Here's how the part is built. I have some questions about the finished solid (model axes, mm). A direction names the side the tool comes from. Round coordinates to 2 decimals unless told otherwise and drop trailing zeros. Loops run counter-clockwise (first coordinate to the right, second up) from the corner with the lowest first, then second, coordinate; pieces in that order, holes last. Notation, with made-up numbers: M -23,2 L 8,2 A15 cw 8,13 Z; hole C -37.75,-2.5 d5. An arc over 180 degrees is marked long. Answer as a JSON object with one key per item and string values.
from build123d import *

# Parameters (mm, degrees)
F1_DEPTH = 64.77
F3_DEPTH = 6.096
F4_R     = 5.860141
F5_DEPTH = 79.248


with BuildPart() as f1:
    # F0 (on Front) → F1 (new body)
    with BuildSketch(Plane.XZ):
        Polygon((32.464709, -14.754961), (0, 14.754961), (-32.464709, 14.754961), (-32.464709, -14.754961), align=None)
    extrude(amount=F1_DEPTH)

    # F2 (on Front) → F3 (join)
    with BuildSketch(Plane.XZ):
        Polygon((-32.523151, -14.200249), (42.600743, -14.200249), (0, 24.277844), (-32.523151, 24.277844), align=None)
    extrude(amount=-F3_DEPTH)

    # F4 (on face) → F5 (cut)
    with BuildSketch(Plane(origin=(0, 0, -14.754961), x_dir=(1, 0, 0), z_dir=(0, 0, -1))):
        with Locations((18.379251, 32.672778)):
            Circle(F4_R)
    extrude(amount=-F5_DEPTH, mode=Mode.SUBTRACT)


solid = f1.part
Item 1: If I drill on L1, parallel to Z at x = -19.5, y = -41; L2, parallel to Y at x = 1, z = 17; L3, parallel to Z at x = 20, y = -44.5, over which ranges is the centre line in solid material (lowest first)? Write a range as from..to.
Solution:
{"L1": "z = -14.75..14.75", "L2": "y = 0..6.1", "L3": "z = -14.75..-3.42"}
Item 2: I want a section at C-C on y = -54.5. List the corners of the cut face in (x, z) for me.
Solution:
{"outline": "M -32.46,-14.75 L 32.46,-14.75 L 0,14.75 L -32.46,14.75 Z"}
Item 3: I want a section at A-A on x = 20. List the corners of the cut face in (y, z) for me, plus the area to 3 significant figures.
Solution:
{"outline": "M -64.77,-14.75 L -38.3,-14.75 L -38.3,-3.42 L -64.77,-3.42 Z; M -27.04,-14.75 L 0,-14.75 L 0,-14.2 L 6.1,-14.2 L 6.1,6.21 L 0,6.21 L 0,-3.42 L -27.04,-3.42 Z", "area": "731 mm2"}
Item 4: For faces 1 (the face through (0, -32, -14.755)), 2 (the face through (16.46, -24.735, -0.207)), 3 (the face through (-16, -32, 14.755)), 4 (the face through (5, 3, -14.2)), 5 (the face through (-8, -64.77, 0)), which set-ups out of +Z, -Z, +X, -X, +Y, -Y let a thin tool reach every point of the face, with its end or its side?
Solution:
{"face 1": "-Z, +X, -X, +Y, -Y", "face 2": "+Z, +X, -Y", "face 3": "+Z, +X, -X, -Y", "face 4": "-Z, +X, -X, +Y", "face 5": "+Z, -Z, +X, -X, -Y"}
Item 5: I want a section at B-B on z = -11.5. List the corners of the cut face in (x, y) for me.
Solution:
{"outline": "M -32.52,0 L -32.46,0 L -32.46,-64.77 L 28.88,-64.77 L 28.88,0 L 39.61,0 L 39.61,6.1 L -32.52,6.1 Z; hole C 18.38,-32.67 d11.72"}
Item 6: For P1, Ø1.8, axis at x = 1.5, y = 1.5, coming from the -Z side; P2, Ø12, axis at y = -26.5, z = 15, coming from the -X side; P3, Ø10, axis at x = -8, y = -24.5, coming from the +Z side; P4, Ø9.5, axis at x = 18.38, y = -32.67, coming from the -Z side (3 decimals), each with a flat end and sliding along its axis, tell me the tip position at first contact or that it passes through.
Solution:
{"P1": "stops at z = -14.2", "P2": "stops at x = -32.46", "P3": "stops at z = 14.75", "P4": "passes through"}
Item 7: I want a section at D-D on x = -17. List the corners of the cut face in (y, z) for me.
Solution:
{"outline": "M -64.77,-14.75 L 0,-14.75 L 0,-14.2 L 6.1,-14.2 L 6.1,24.28 L 0,24.28 L 0,14.75 L -64.77,14.75 Z"}
